from build123d import *

# Parameters (mm, degrees)
BOSS_EXTRUDE1_DEPTH = 5
SKETCH2_R           = 2.5
SKETCH2_W           = 10
SKETCH2_H           = 20
CUT_EXTRUDE1_DEPTH  = 5
SKETCH3_W           = 20
SKETCH3_H           = 5
CUT_EXTRUDE2_DEPTH  = 5


with BuildPart() as part:
    # Sketch1 → Boss-Extrude1 (new body)
    with BuildSketch(Plane(origin=(0, 0, 0), x_dir=(0, 0, -1), z_dir=(1, 0, 0))):
        Polygon((65, 35), (65, 25), (60, 25), (60, 5), (65, 5), (65, -5), (60, -5), (60, -25), (65, -25), (65, -35), (60, -35), (45, -35), (45, -40), (25, -40), (25, -35), (10, -35), (10, -40), (-10, -40), (-10, -35), (-25, -35), (-25, -40), (-45, -40), (-45, -35), (-60, -35), (-65, -35), (-65, -25), (-60, -25), (-60, -5), (-65, -5), (-65, 5), (-60, 5), (-60, 25), (-65, 25), (-65, 35), (-60, 35), (-45, 35), (-45, 40), (-25, 40), (-25, 35), (-10, 35), (-10, 40), (10, 40), (10, 35), (25, 35), (25, 40), (45, 40), (45, 35), (60, 35), align=None)
    extrude(amount=BOSS_EXTRUDE1_DEPTH)

    # Sketch2 → Cut-Extrude1 (cut)
    with BuildSketch(Plane(origin=(0, 0, 0), x_dir=(0, 0, -1), z_dir=(1, 0, 0))):
        with Locations((23, 6)):
            Circle(SKETCH2_R)
        with Locations(Location((23, -6, 0), (0, 0, 180))):
            Circle(SKETCH2_R)
        with Locations((-23, -6)):
            Circle(SKETCH2_R)
        with Locations(Location((-23, 6, 0), (0, 0, 180))):
            Circle(SKETCH2_R)
        Rectangle(SKETCH2_W, SKETCH2_H)
    extrude(amount=CUT_EXTRUDE1_DEPTH, mode=Mode.SUBTRACT)

    # Sketch3 → Cut-Extrude2 (cut)
    with BuildSketch(Plane(origin=(5, 0, 0), x_dir=(0, 0, -1), z_dir=(1, 0, 0))):
        with Locations((30, -17.5)):
            Rectangle(SKETCH3_W, SKETCH3_H)
        with Locations((-30, -17.5)):
            Rectangle(SKETCH3_W, SKETCH3_H)
    extrude(amount=-CUT_EXTRUDE2_DEPTH, mode=Mode.SUBTRACT)


solid = part.part
Check sheet for the modelled part. Datum: model origin and axes. Units: mm. A direction names the side the tool comes from. Round coordinates to 2 decimals unless told otherwise and drop trailing zeros. Order: outer loops, then holes, each group sorted by start corner. A loop starts at its lowest first (then second) coordinate and runs counter-clockwise, first axis right, second up. Notation, with made-up numbers: M 25.5,34.5 L 44.5,34.5 A18 ccw 44.5,57.5 Z; hole C -13,87 d9. An arc over 180 degrees is marked long. One line per item, written item: value. Start each with the question number.
1. Scan lines: line 1 along Y through (x, z) = (3.9, 23); line 2 along Y through (x, z) = (4.2, -34); line 3 along Y through (x, z) = (2, 4.5). Record each from-to range of solid material in increasing order.
2. Section check C-C on y = 11.5. Enter the section's corners in (x, z).
3. Section check A-A on z = 23. Enter the section's corners in (x, y), and give its area (3 significant figures).
4. Section check D-D on x = 4.2. Give the number of separate pieces and of enclosed holes in the cut face, and give its area (3 significant figures).
5. Gauge pin test, flat ends, axial feed: P1, Ø3, axis at x = 3.5, y = -22.5, coming from the -Z side; P2, Ø1.5, axis at x = 3.5, y = 15, coming from the +Z side; P3, Ø2.5, axis at x = 1.5, y = -37, coming from the +Z side. Record the tip position at first contact, or that the pin passes through.
6. Section check B-B on z = -1.5. Enter the section's corners in (x, y).
7. Release check for a two-part mould opening along Z. For faces 1 (the flat face through (2, -35, 17)), 2 (the flat face through (2, 5, -62)), 3 (the flat face through (3, -20, -30)), 4 (the flat face through (2, 0, 65)) record: released by +Z, released by -Z, zero draft, split by the parting line, or undercut.
8. Access from +Z, -Z, +X, -X, +Y, -Y to the whole of each face (thin tool, end or side, straight path). Record for faces 5 (the flat face through (2, -15, 60)), 6 (the flat face through (2, 35, -17)), 7 (the flat face through (2, -38, 45)), 8 (the flat face through (2, -15, -60)), 9 (the flat face through (2, -10, 0)).
Results found:
1. line 1: -35 to -20, -15 to -8.5, -3.5 to 3.5, 8.5 to 35
1. line 2: -40 to -20, -15 to 40
1. line 3: -40 to -10, 10 to 40
2. outline: M 0,-60 L 5,-60 L 5,60 L 0,60 Z
3. outline: M 0,-35 L 5,-35 L 5,-20 L 0,-20 Z; M 0,-15 L 5,-15 L 5,-8.5 L 0,-8.5 Z; M 0,-3.5 L 5,-3.5 L 5,3.5 L 0,3.5 Z; M 0,8.5 L 5,8.5 L 5,35 L 0,35 Z
3. area: 275 mm^2
4. separate pieces: 1
4. enclosed holes: 7
4. area: 8,820 mm^2
5. P1: z = -60
5. P2: z = 60
5. P3: z = 45
6. outline: M 0,-40 L 5,-40 L 5,-10 L 0,-10 Z; M 0,10 L 5,10 L 5,40 L 0,40 Z
7. face 1: undercut
7. face 2: zero draft
7. face 3: undercut
7. face 4: released by +Z
8. face 5: +Z, +X, -X
8. face 6: +X, -X, +Y
8. face 7: +Z, +X, -X, -Y
8. face 8: -Z, +X, -X
8. face 9: +X, -X
